Drawing for the job (mm, zero at the part's lowest x, y, z). Round coordinates to 2 decimals unless told otherwise and drop trailing zeros. Loops run counter-clockwise (first coordinate to the right, second up) from the corner with the lowest first, then second, coordinate; pieces in that order, holes last. Notation, with made-up numbers: (64, 35) - (112, 35) arc R31 cw to (112, 72) - close; hole circle Ø1 at (75.5, 37). An arc over 180 degrees is marked (long way). Put each result on its own line as item: value.
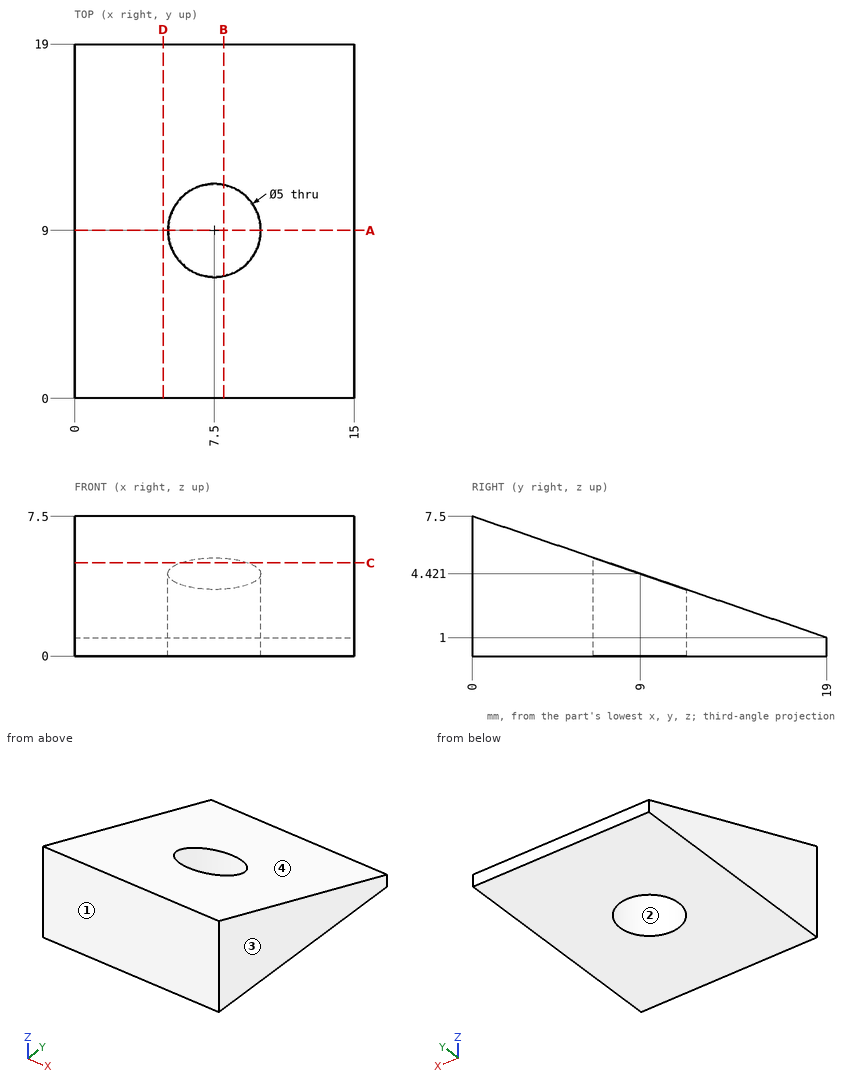
1. Pin check, flat tips, straight feed: P1, Ø1, axis at x = 13, y = 8, coming from the +Z side; P2, Ø5, axis at x = 12.5, y = 7.5, coming from the +Z side; P3, Ø4.5, axis at x = 7.5, y = 9, coming from the -Z side. Stop position of each tip, or through.
A:
P1: stops at z = 4.93
P2: stops at z = 5.79
P3: passes through
2. Two-plate mould, pull along Y, no slides. Class the marked faces 1, 2, 3 and 4: pulls with the +Y half, pulls with the -Y half, needs draft (parallel to the pull), parting line crosses it, or undercut.
A:
face 1: pulls with the -Y half
face 2: undercut
face 3: needs draft
face 4: pulls with the +Y half
3. Band-saw the part on C-C (z = 5). List the corners of the cut face in (x, y), plus the area to 3 significant figures.
A:
outline: (0, 0) - (15, 0) - (15, 7.31) - (9.34, 7.31) arc R2.5 cw to (5.66, 7.31) - (0, 7.31) - close
area: 108 mm²
4. Probe line 1 along X through (y, z) = (9, 1.45); line 2 along X through (y, z) = (9.5, 3.75); line 3 along Z through (x, y) = (14, 8). List the from-to ranges inside material, lowest first. Write a range as [from, to].
A:
line 1: x = [0, 5], [10, 15]
line 2: x = [0, 5.05], [9.95, 15]
line 3: z = [0, 4.76]
5. Band-saw the part on D-D (x = 4.75). List the corners of the cut face in (y, z).
A:
outline: (0, 0) - (19, 0) - (19, 1) - (0, 7.5) - close
6. Band-saw the part on B-B (x = 8). List the corners of the cut face in (y, z), plus the area to 3 significant figures.
A:
outline: (0, 0) - (6.55, 0) - (6.55, 5.26) - (0, 7.5) - close; (11.45, 0) - (19, 0) - (19, 1) - (11.45, 3.58) - close
area: 59.1 mm²
7. Band-saw the part on A-A (y = 9). List the corners of the cut face in (x, z).
A:
outline: (0, 0) - (5, 0) - (5, 4.42) - (0, 4.42) - close; (10, 0) - (15, 0) - (15, 4.42) - (10, 4.42) - close
